Job drawing, mm, ordinate dimensions from the low corner. One solid piece. A direction names the side the tool comes from. Round coordinates to 2 decimals unless told otherwise and drop trailing zeros. Order: outer loops, then holes, each group sorted by start corner. A loop starts at its lowest first (then second) coordinate and runs counter-clockwise, first axis right, second up. Notation, with made-up numbers: (-11, 86) - (40, 86) arc R24 ccw to (40, 105) - close; hole circle Ø4 at (31.25, 77). An arc over 180 degrees is marked (long way). Write each question's results on one line, items separated by ' | '. Start each with the question number.
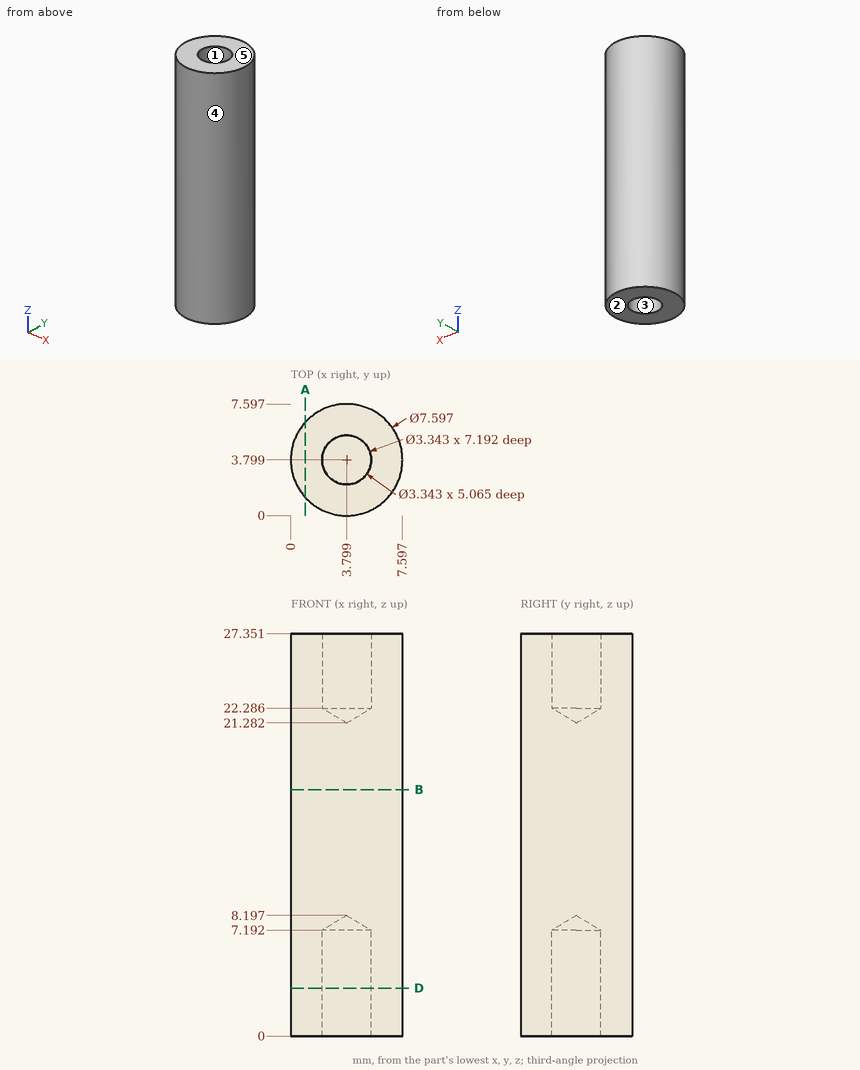
1. Cut at D-D (z = 3.25). List the corners of the cut face in (x, y).
2. Wall check: line 1 (Y direction, x = 3.75, z = 5.5); line 2 (Y direction, x = 4.5, z = 5) (1 decimal); line 3 (X direction, y = 4.25, z = 7.5) (1 decimal). Give the ranges that are in metal, low to high. Write a range as from..to.
3. Cut at B-B (z = 16.75). List the corners of the cut face in (x, y).
4. Flat gauge pins, fed straight in: pin 1 Ø3 at (x, z) = (1, 3.5) entering from -Y; pin 2 Ø3 at (y, z) = (2, 11) entering from -X; pin 3 Ø3 at (x, z) = (6.5, 18.5) entering from +Y. Where does each tip first touch, or does it go through?
5. Mould opens along Y. For the marked faces 3, 4 and 5 say: pulls with the +Y half, pulls with the -Y half, needs draft (parallel to the pull), parting line crosses it, or undercut.
6. Cut at A-A (x = 1). List the corners of the cut face in (y, z).
7. 3-axis set-ups, long thin cutter, end or side, ignore diameter. For the marked faces 1 and 2: which of +Z, -Z, +X, -X, +Y, -Y reach the whole face in a straight line?
A:
1) outline: circle Ø7.6 at (3.8, 3.8); hole circle Ø3.34 at (3.8, 3.8)
2) line 1: y = 0..2.13, 5.47..7.6 | line 2: y = 0.1..2.3, 5.3..7.5 | line 3: x = 0..2.7, 4.9..7.6
3) outline: circle Ø7.6 at (3.8, 3.8)
4) pin 1: stops at y = 0.23 | pin 2: stops at x = 0.01 | pin 3: stops at y = 7.4
5) face 3: undercut | face 4: parting line crosses it | face 5: needs draft
6) outline: (1.23, 0) - (6.37, 0) - (6.37, 27.35) - (1.23, 27.35) - close
7) face 1: +Z | face 2: -Z, +X, -X, +Y, -Y
